The model under review builds one solid part; all positions refer to its coordinate system, in mm. Round coordinates to 2 decimals unless told otherwise and drop trailing zeros. Write each loop counter-clockwise with the first axis right and the second up, starting at its lowest first coordinate (ties: lowest second). Pieces come first, ordered by that corner, then holes. Notation, with made-up numbers: (-35, 85) -> (-28, 85) arc R18 ccw to (-28, 108) -> close; hole circle Ø8 at (65, -27). An arc over 180 degrees is marked (long way). Return JSON: item names as keys, results as strings. Group by question number.
1. Clearance check with a flat-ended pin moving along its axis: P1, Ø5, axis at x = -18, z = -13.5, coming from the -Y side. State where the tip first meets the part, or that it passes through.
2. Take a section at A-A, the plane x = 19. Write out the cut boundary in (y, z) (3 decimals), then the cut area to 3 significant figures.
3. Take a section at B-B, the plane z = -8.25. Write out the cut boundary in (x, y) (3 decimals), then the cut area to 3 significant figures.
4. For line 1 along X through (y, z) = (0.9, 28) (3 decimals); line 2 along X through (y, z) = (0.7, -8.25) (3 decimals); line 3 along Z through (x, y) = (-14, 0.65), list the stretches that pass through material, from the lowest coordinate up. Write a range as from..to.
from build123d import *

# Parameters (mm, degrees)
SKETCH_1_W          = 46
SKETCH_1_H          = 62
EXTRUDE_1_DEPTH     = 2
SKETCH_2_R          = 1.525
CUT_EXTRUDE_1_DEPTH = 2
SKETCH_3_R          = 1.525
CUT_EXTRUDE_2_DEPTH = 2
FILLET_1_R          = 3


with BuildPart() as part:
    # 草图1 → 凸台-拉伸1 (new body)
    with BuildSketch(Plane(origin=(0, 0, 0), x_dir=(1, 0, 0), z_dir=(0, 1, 0))):
        Rectangle(SKETCH_1_W, SKETCH_1_H)
    extrude(amount=EXTRUDE_1_DEPTH)

    # 草图2 → 切除-拉伸1 (cut)
    with BuildSketch(Plane.XZ):
        with Locations(Location((19, -8.25, 0), (0, 0, 270))):
            Circle(SKETCH_2_R)
        with Locations(Location((-19, -8.25, 0), (0, 0, 270))):
            Circle(SKETCH_2_R)
    extrude(amount=-CUT_EXTRUDE_1_DEPTH, mode=Mode.SUBTRACT)

    # 草图3 → 切除-拉伸2 (cut)
    with BuildSketch(Plane.XZ):
        with Locations(Location((5, 28, 0), (0, 0, 270))):
            Circle(SKETCH_3_R)
        with Locations(Location((-15, 28, 0), (0, 0, 270))):
            Circle(SKETCH_3_R)
    extrude(amount=-CUT_EXTRUDE_2_DEPTH, mode=Mode.SUBTRACT)

    # 圆角1
    fillet_1_edges = [part.edges().sort_by_distance(p)[0] for p in [
        (23, 1, 31),
        (-23, 1, 31),
        (-23, 1, -31),
        (23, 1, -31),
    ]]
    fillet(fillet_1_edges, radius=FILLET_1_R)


solid = part.part
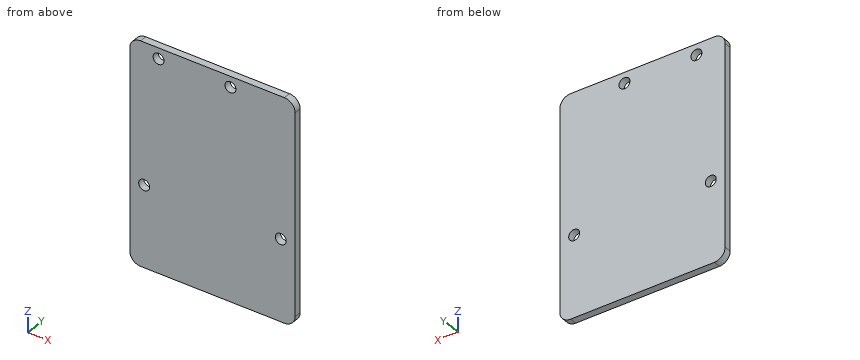
Output:
{
 "1": {"P1": "stops at y = 0"},
 "2": {"outline": "(0, -31) -> (2, -31) -> (2, -9.775) -> (0, -9.775) -> close; (0, -6.725) -> (2, -6.725) -> (2, 31) -> (0, 31) -> close", "area": "118 mm^2"},
 "3": {"outline": "(-23, 0) -> (-20.525, 0) -> (-20.525, 2) -> (-23, 2) -> close; (-17.475, 0) -> (17.475, 0) -> (17.475, 2) -> (-17.475, 2) -> close; (20.525, 0) -> (23, 0) -> (23, 2) -> (20.525, 2) -> close", "area": "79.8 mm^2"},
 "4": {"line 1": "x = -23..-16.525, -13.475..3.475, 6.525..23", "line 2": "x = -23..-20.525, -17.475..17.475, 20.525..23", "line 3": "z = -31..26.85, 29.15..31"}
}
